The model under review builds one solid part; all positions refer to its coordinate system, in mm. Face numbers are marked on the shaded views. Coordinates: 2 decimals unless noted, no trailing zeros. Write each loop counter-clockwise with the first axis right and the second up, starting at its lowest first coordinate (ties: lowest second). Pieces come first, ordered by that corner, then holes.
1) For line 1 (X direction, y = 15.5, z = 0); line 2 (Z direction, x = 1, y = 68); line 3 (X direction, y = 23, z = 4.5), list the stretches that pass through material, from the lowest coordinate up.
2) Add section A-A, the plane y = 89.5. State the section outline as (x, z) points, then the cut area to 3 significant figures.
3) For P1, Ø6, axis at x = -1.5, z = -7.5, coming from the -Y side; P2, Ø10, axis at y = 18, z = 10, coming from the +X side; P3, Ø4, axis at y = 21, z = 4.5, coming from the -X side, all flat-tipped, find the tip position at first contact; note any pin that passes through.
4) Mouldability with a two-part tool opening along Z and no side actions: class the marked faces 1 and 2 as released by +Z, released by -Z, zero draft, split by the parting line, or undercut.
5) Add section B-B, the plane y = 28. State the section outline as (x, z) points.
from build123d import *

# Parameters (mm, degrees)
CORTAR_EXTRUIR6_START = 40
CROQUIS3_RX           = 4.5
CROQUIS3_RY           = 4
CORTAR_EXTRUIR6_DEPTH = 143
REDONDEO5_R           = 1.5


with BuildPart() as part:
    # Croquis2 → Revolución2 (revolve)
    with BuildSketch(Plane.XY, mode=Mode.PRIVATE) as revoluci_n2_sk:
        with BuildLine():
            Line((-15.5, 100), (-15.5, 90.866072441))
            ThreePointArc((-15.5, 90.866072441), (-14.482138299, 82.547634192), (-15.5, 74.229195944))
            Line((-15.5, 74.229195944), (-15.5, 73.866072441))
            ThreePointArc((-15.5, 73.866072441), (-14.482138299, 65.547634192), (-15.5, 57.229195944))
            Line((-15.5, 57.229195944), (-15.5, 56.866072441))
            ThreePointArc((-15.5, 56.866072441), (-14.482138299, 48.547634192), (-15.5, 40.229195944))
            Line((-15.5, 40.229195944), (-15.5, 39.866072441))
            ThreePointArc((-15.5, 39.866072441), (-14.482138299, 31.547634192), (-15.5, 23.229195944))
            Line((-15.5, 23.229195944), (-15.5, 0))
            Line((-15.5, 0), (-14, 0))
            Line((-14, 0), (-14, 23.047634192))
            ThreePointArc((-14, 23.047634192), (-12.982138299, 31.547634192), (-14, 40.047634192))
            ThreePointArc((-14, 40.047634192), (-12.982138299, 48.547634192), (-14, 57.047634192))
            ThreePointArc((-14, 57.047634192), (-12.982138299, 65.547634192), (-14, 74.047634192))
            ThreePointArc((-14, 74.047634192), (-12.982138299, 82.547634192), (-14, 91.047634192))
            Line((-14, 91.047634192), (-14, 100))
            ThreePointArc((-14, 100), (-9.956223855, 110.259142264), (0, 115))
            Line((0, 115), (0, 116.496437055))
            Line((0, 116.496437055), (-0.103325416, 116.496437055))
            ThreePointArc((-0.103325416, 116.496437055), (-11.052806757, 111.28261964), (-15.5, 100))
        make_face()
    revolve(revoluci_n2_sk.sketch.rotate(Axis((0, 0, 0), (0, 1, 0)), 270), axis=Axis((0, 0, 0), (0, 1, 0)))

    # Croquis3 → Cortar-Extruir6 (cut)
    with BuildSketch(Plane(origin=(0, 0, 0), x_dir=(1, 0, 0), z_dir=(0, 1, 0)).offset(CORTAR_EXTRUIR6_START)):
        with Locations(Location((0, 0), (0, 0, -90))):
            Ellipse(CROQUIS3_RX, CROQUIS3_RY)
    extrude(amount=CORTAR_EXTRUIR6_DEPTH, mode=Mode.SUBTRACT)

    # Redondeo5
    redondeo5_edges = [part.edges().sort_by_distance(p)[0] for p in [
        (0, 74.229195944, 15.5),
        (0, 73.866072441, 15.5),
        (0, 57.229195944, 15.5),
        (0, 56.866072441, 15.5),
        (0, 40.229195944, 15.5),
        (0, 39.866072441, 15.5),
        (0, 23.229195944, 15.5),
    ]]
    fillet(redondeo5_edges, radius=REDONDEO5_R - 0.0001)  # a hair under: the kernel refuses the full size


solid = part.part
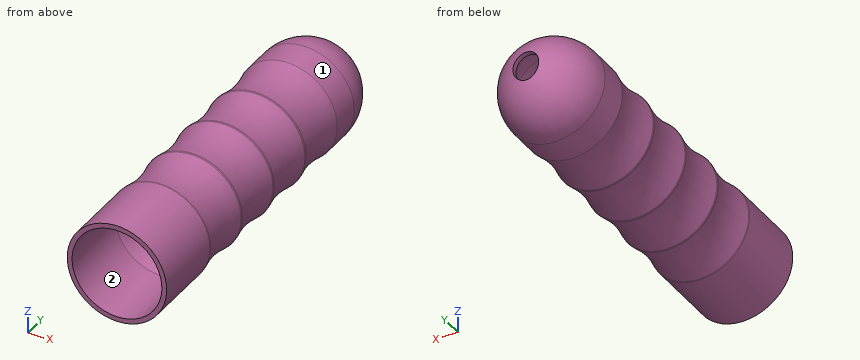
Geometry results:
1. line 1: x = -15.5 to -14, 14 to 15.5
1. line 2: z = -14.54 to -13.03, 13.03 to 14.54
1. line 3: x = -14.83 to -13.26, 13.26 to 14.83
2. outline: circle Ø30.38 at (0, 0); hole circle Ø27.32 at (0, 0)
2. area: 139 mm2
3. P1: stops at y = 109.46
3. P2: stops at x = 14.67
3. P3: stops at x = -15.3
4. face 1: split by the parting line
4. face 2: undercut
5. outline: circle Ø29.33 at (0, 0); hole circle Ø26.31 at (0, 0)
